Autodesk Inventor part; units mm, degrees
ref_plane "YZ Plane" through (0, 0, 0) normal (1, 0, 0) x (0, 1, 0)
ref_plane "XZ Plane" through (0, 0, 0) normal (0, 1, 0) x (-1, 0, 0)
ref_plane "XY Plane" through (0, 0, 0) normal (0, 0, 1) x (1, 0, 0)
sketch "Sketch1" plane through (0, 0, 0) normal (0, 1, 0) x (-1, 0, 0)
  line L0 (0, 0) -> (30, 0)
  line L1 (30, 0) -> (30, -80)
  line L2 (30, -80) -> (0, -80)
  line L3 (0, -80) -> (0, 0)
  line L4 (30, -80) -> (80, -80)
  line L5 (80, -80) -> (80, -50)
  line L6 (80, -50) -> (30, -50)
  line L7 (30, -50) -> (30, -80)
  dimension "d0" = 30
  dimension "d1" = 80
  dimension "d2" = 50
  dimension "d3" = 30
extrude "Extrusion1" add sketch "Sketch1" along normal blind 10
sketch "Sketch2" plane through (0, 10, 0) normal (0, 1, 0) x (1, 0, 0)
  line L0 (-30, 0) -> (0, 0)
  line L1 (-30, 0) -> (-20, 0)
  line L2 (-20, 0) -> (-20, 50)
  line L3 (-20, 50) -> (-30, 50)
  line L4 (-30, 50) -> (-30, 0)
  line L5 (-80, 80) -> (-80, 50)
  line L6 (-80, 50) -> (-20, 50)
  line L7 (-20, 50) -> (-20, 60)
  line L8 (-20, 60) -> (-80, 60)
  line L9 (-80, 60) -> (-80, 50)
  line L10 (-80, 80) -> (0, 80)
  line L11 (0, 80) -> (0, 70)
  line L12 (0, 70) -> (-80, 70)
  line L13 (-80, 70) -> (-80, 80)
  line L14 (0, 70) -> (-10, 70)
  line L15 (-10, 70) -> (-10, 0)
  line L16 (-10, 0) -> (0, 0)
  line L17 (0, 0) -> (0, 70)
  dimension "d6" = 10
  dimension "d7" = 10
  dimension "d8" = 80
  dimension "d9" = 10
  dimension "d10" = 10
extrude "Extrusion2" add sketch "Sketch2" along normal blind 20 contours L4 L3 L2 L0 | L6 L5 L8 L7 L3 | L15 L12 L17 L0 | L12 L5 L10 L11
fillet "Fillet1" radius 10 6 edges at (-30, 15, -50) (-30, 15, 0) (-80, 15, -50) (-80, 15, -80) (0, 15, -80) (0, 15, 0)
fillet "Fillet2" radius 2 12 edges at (-55, 30, -50) (-77.0711, 30, -52.9289) (-30, 30, -25) (-27.0711, 30, -2.9289) (-77.0711, 30, -77.0711) (-2.9289, 30, -77.0711) (-2.9289, 30, -2.9289) (-40, 30, -80) (-45, 30, -70) (-50, 30, -60) (-10, 30, -35) (-20, 30, -30)
properties part number "TSU_Corner_Top_Clamp"
The model under review builds one solid part; all positions refer to its coordinate system, in mm. A direction names the side the tool comes from. Give positions to 0.01 mm unless a question says otherwise; leave off trailing zeros. Write each loop counter-clockwise with the first axis right and the second up, starting at its lowest first coordinate (ties: lowest second). Pieces come first, ordered by that corner, then holes. Notation, with made-up numbers: M 54,89 L 72,89 A18 cw 72,111 Z; hole C -30,-22 d9. An arc over 180 degrees is marked long. Write item = value, one per line. Start each with the question number.
Q1. Mouldability with a two-part tool opening along Z and no side actions: class faces 4 (the face through (-20.6, 29.43, -30.42)), 5 (the face through (-44.5, 29.4, -70.57)), 6 (the face through (-3.01, 14.2, -2.85)), 7 (the face through (-50.42, 29.43, -59.4)) as released by +Z, released by -Z, zero draft, split by the parting line, or undercut.
Q2. We need section A-A (y = 19). State the section outline as (x, z) points, plus the area to 3 significant figures.
Q3. Clearance check with flat-ended pins moving along their axes: pin 1 (1.5 mm diameter, centred on x = -28.5, y = 4.5, fed in from +Z); pin 2 (8.5 mm diameter, centred on y = 20.5, z = -28, fed in from -X); pin 3 (14.5 mm diameter, centred on x = -62.5, y = 20, fed in from +Z). State where each tip first meets the part, or that it passes through.
Q4. We need section D-D (y = 4.5). State the section outline as (x, z) points.
Q5. We need section C-C (x = -13). State the section outline as (y, z) points.
Q6. For line 1 (Z direction, x = -52.5, y = 22); line 2 (X direction, y = 21, z = -18); line 3 (Z direction, x = -54, y = 7), list the stretches that pass through material, from the lowest coordinate up.
Q7. Machinability: for faces 1 (the face through (-55, 14, -50)), 2 (the face through (-29.4, 29.43, -24.79)), 3 (the face through (-20, 19, -30)), which of the approach directions +Z, -Z, +X, -X, +Y, -Y give a long, thin tool a straight path to every point of the face, cutting with its end or side? Answer none if there is none.
Q8. We need section B-B (z = -17.5). State the section outline as (x, y) points.
Result set:
q1.face_4 = zero draft
q1.face_5 = undercut
q1.face_6 = released by +Z
q1.face_7 = undercut
q2.outline = M -80,-70 A10 ccw -70,-80 L -10,-80 A10 ccw 0,-70 L 0,-10 A10 ccw -10,0 L -10,-70 Z; M -80,-60 L -20,-60 L -20,0 A10 ccw -30,-10 L -30,-40 A10 cw -40,-50 L -70,-50 A10 ccw Z
q2.area = 2,510 mm2
q3.pin_1 = -3.68
q3.pin_2 = -30
q3.pin_3 = -50
q4.outline = M -80,-70 A10 ccw -70,-80 L -10,-80 A10 ccw 0,-70 L 0,-10 A10 ccw -10,0 L -20,0 A10 ccw -30,-10 L -30,-40 A10 cw -40,-50 L -70,-50 A10 ccw -80,-60 Z
q5.outline = M 0,-80 L 28,-80 A2 ccw 30,-78 L 30,-72 A2 ccw 28,-70 L 10,-70 L 10,0 L 0,0 Z
q6.line_1 = -80 to -70, -60 to -50
q6.line_2 = -30 to -20, -10 to 0
q6.line_3 = -80 to -50
q7.face_1 = +Z, -X, +Y, -Y
q7.face_2 = +Z, -X, +Y
q7.face_3 = +Z, +Y
q8.outline = M -30,0 L 0,0 L 0,28 A2 ccw -2,30 L -8,30 A2 ccw -10,28 L -10,10 L -20,10 L -20,28 A2 ccw -22,30 L -28,30 A2 ccw -30,28 Z
